```python
from build123d import *

# Parameters (mm, degrees)
SKETCH_W     = 150
SKETCH_H     = 56
SKETCH_R     = 8
SKETCH_W_2   = 73
SKETCH_H_2   = 25
PAD_DEPTH    = 2
PAD001_DEPTH = 5
SKETCH002_R  = 1.5
POCKET_DEPTH = 5
FILLET_R     = 1


with BuildPart() as part:
    # Sketch → Pad (new body)
    with BuildSketch(Plane.XY):
        with Locations((75, 28)):
            Rectangle(SKETCH_W, SKETCH_H)
        with Locations((17.5, 16.5)):
            Circle(SKETCH_R, mode=Mode.SUBTRACT)
        with Locations((17.5, 39.5)):
            Circle(SKETCH_R, mode=Mode.SUBTRACT)
        with Locations((132.5, 16.5)):
            Circle(SKETCH_R, mode=Mode.SUBTRACT)
        with Locations((132.5, 39.5)):
            Circle(SKETCH_R, mode=Mode.SUBTRACT)
        with Locations((75, 28)):
            Rectangle(SKETCH_W_2, SKETCH_H_2, mode=Mode.SUBTRACT)
    extrude(amount=PAD_DEPTH)

    # Sketch001 (on Face14 of Pad) → Pad001 (join)
    with BuildSketch(Plane.XY.offset(2)):
        Polygon((38.5, 15.5), (111.5, 15.5), (116.5, 15.5), (116.5, 8.5), (109.5, 8.5), (109.5, 14.5), (33.5, 14.5), (33.5, 45.5), (111.5, 45.5), (116.5, 45.5), (116.5, 40.5), (111.5, 40.5), (38.5, 40.5), align=None)
    extrude(amount=PAD001_DEPTH)

    # Sketch002 (on Face5 of Pad001) → Pocket (cut)
    with BuildSketch(Plane.XY.offset(2)):
        with Locations((3, 53)):
            Circle(SKETCH002_R)
        with Locations((147, 53)):
            Circle(SKETCH002_R)
        with Locations((3, 3)):
            Circle(SKETCH002_R)
        with Locations((147, 3)):
            Circle(SKETCH002_R)
    extrude(amount=-POCKET_DEPTH, mode=Mode.SUBTRACT)

    # Fillet
    fillet_edges = [part.edges().sort_by_distance(p)[0] for p in [
        (0, 0, 1),
        (150, 0, 1),
        (150, 56, 1),
        (0, 56, 1),
    ]]
    fillet(fillet_edges, radius=FILLET_R)


solid = part.part
```
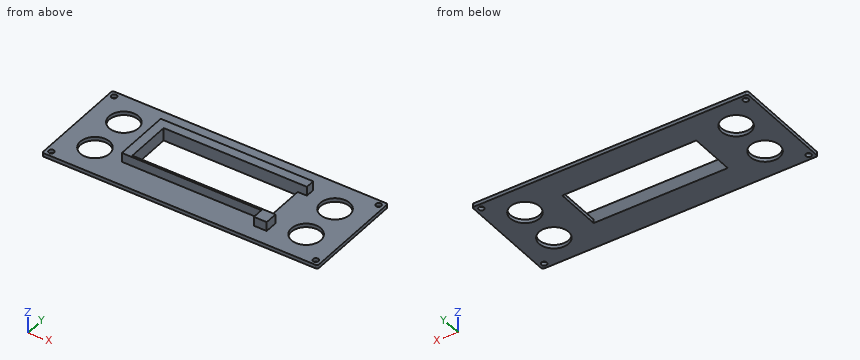
Source: CAD feature listing. Evaluate the final solid. Frame: model axes, mm. Coordinates: 2 decimals unless noted, no trailing zeros. Write each loop counter-clockwise with the first axis right and the second up, starting at its lowest first coordinate (ties: lowest second). Pieces come first, ordered by that corner, then holes. Notation, with made-up numbers: (49.25, 88.5) -> (82.25, 88.5) arc R10 ccw to (82.25, 100.5) -> close; hole circle Ø7 at (-8.75, 39). An arc over 180 degrees is marked (long way). Return JSON: item names as keys, results as strings. Group by question number.
1) Section query A-A, the plane x = 147. Return loops of the section in (y, z), plus the area to 3 significant figures.
2) Ray query, line 1 along Y through (x, z) = (147, 1.5); line 2 along Y through (x, z) = (132.5, 0.85); line 3 along Y through (x, z) = (67.5, 5). Return the intervals inside material, ascending.
3) Section query B-B, the plane y = 53. Return loops of the section in (x, z).
4) Contact query for flat-ended pins moving along their axis: P1, Ø4, axis at x = 113, z = 5.5, coming from the -Y side; P2, Ø1.5, axis at x = 88, z = 4, coming from the -Y side; P3, Ø2.5, axis at y = 42.5, z = 5.5, coming from the +X side. Output: stop coordinate, or through.
5) Section query D-D, the plane z = 5.75. Return loops of the section in (x, y), plus the area to 3 significant figures.
6) Section query C-C, the plane x = 105. Return loops of the section in (y, z), plus the area to 3 significant figures.
From the geometry:
{
 "1": {"outline": "(0, 0) -> (1.5, 0) -> (1.5, 2) -> (0, 2) -> close; (4.5, 0) -> (51.5, 0) -> (51.5, 2) -> (4.5, 2) -> close; (54.5, 0) -> (56, 0) -> (56, 2) -> (54.5, 2) -> close", "area": "100 mm²"},
 "2": {"line 1": "0 to 1.5, 4.5 to 51.5, 54.5 to 56", "line 2": "0 to 8.5, 24.5 to 31.5, 47.5 to 56", "line 3": "14.5 to 15.5, 40.5 to 45.5"},
 "3": {"outline": "(0, 0) -> (1.5, 0) -> (1.5, 2) -> (0, 2) -> close; (4.5, 0) -> (145.5, 0) -> (145.5, 2) -> (4.5, 2) -> close; (148.5, 0) -> (150, 0) -> (150, 2) -> (148.5, 2) -> close"},
 "4": {"P1": "y = 8.5", "P2": "y = 14.5", "P3": "x = 116.5"},
 "5": {"outline": "(33.5, 14.5) -> (109.5, 14.5) -> (109.5, 8.5) -> (116.5, 8.5) -> (116.5, 15.5) -> (38.5, 15.5) -> (38.5, 40.5) -> (116.5, 40.5) -> (116.5, 45.5) -> (33.5, 45.5) -> close", "area": "665 mm²"},
 "6": {"outline": "(0, 0) -> (15.5, 0) -> (15.5, 7) -> (14.5, 7) -> (14.5, 2) -> (0, 2) -> close; (40.5, 0) -> (56, 0) -> (56, 2) -> (45.5, 2) -> (45.5, 7) -> (40.5, 7) -> close", "area": "92.0 mm²"}
}
